Design review of the part built by this model. Coordinates are the model's own, in mm. Give positions to 0.01 mm unless a question says otherwise; leave off trailing zeros. Loops run counter-clockwise (first coordinate to the right, second up) from the corner with the lowest first, then second, coordinate; pieces in that order, holes last. Notation, with made-up numbers: (39, 77.5) -> (92, 77.5) arc R16 cw to (92, 102.5) -> close; hole circle Ø4 at (78.5, -28). An arc over 180 degrees is marked (long way). Answer as CSV lines item,"result".
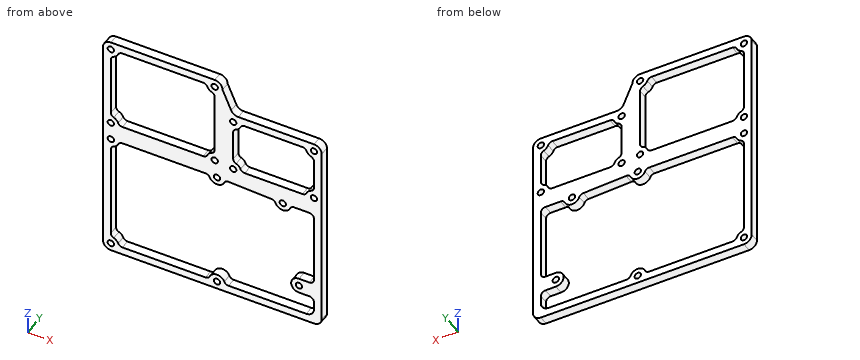
from build123d import *

# Parameters (mm, degrees)
SKETCH2_R                = 3.375
SKETCH2_R_2              = 1.375
PART_SCREWHOLES_DEPTH    = 4
PART_SCREWHOLES_2_DEPTH  = 4
PART_SCREWHOLES_3_DEPTH  = 4
PART_SCREWHOLES_4_DEPTH  = 4
PART_SCREWHOLES_5_DEPTH  = 4
PART_SCREWHOLES_6_DEPTH  = 4
PART_SCREWHOLES_7_DEPTH  = 4
PART_SCREWHOLES_8_DEPTH  = 4
PART_SCREWHOLES_9_DEPTH  = 4
PART_SCREWHOLES_10_DEPTH = 4
PART_SCREWHOLES_11_DEPTH = 4
PART_SCREWHOLES_12_DEPTH = 4
PART_SCREWHOLES_13_DEPTH = 4
PART_SCREWHOLES_14_DEPTH = 4
FRAME_START              = -4
SKETCH3_R                = 1.375
FRAME_DEPTH              = 4
GENERAL_ROUNDING_2MM_R   = 2


with BuildPart() as part:
    # Sketch2 → Part screwholes (new body)
    with BuildSketch(Plane(origin=(0, 0, 0), x_dir=(1, 0, 0), z_dir=(0, 1, 0))):
        with Locations(Location((-46, 51, 0), (0, 0, 270))):
            Circle(SKETCH2_R)
        with Locations(Location((-46, 51, 0), (0, 0, 270))):
            Circle(SKETCH2_R_2, mode=Mode.SUBTRACT)
    extrude(amount=PART_SCREWHOLES_DEPTH)



with BuildPart() as body_2:
    # Sketch2 → Part screwholes 2 (new body)
    with BuildSketch(Plane(origin=(0, 0, 0), x_dir=(1, 0, 0), z_dir=(0, 1, 0))):
        with Locations(Location((0, 51, 0), (0, 0, 270))):
            Circle(SKETCH2_R)
        with Locations(Location((0, 51, 0), (0, 0, 270))):
            Circle(SKETCH2_R_2, mode=Mode.SUBTRACT)
    extrude(amount=PART_SCREWHOLES_2_DEPTH)


with BuildPart() as body_3:
    # Sketch2 → Part screwholes 3 (new body)
    with BuildSketch(Plane(origin=(0, 0, 0), x_dir=(1, 0, 0), z_dir=(0, 1, 0))):
        with Locations(Location((0, 0, 0), (0, 0, 270))):
            Circle(SKETCH2_R)
        with Locations(Location((0, 0, 0), (0, 0, 270))):
            Circle(SKETCH2_R_2, mode=Mode.SUBTRACT)
    extrude(amount=PART_SCREWHOLES_3_DEPTH)


with BuildPart() as body_4:
    # Sketch2 → Part screwholes 4 (new body)
    with BuildSketch(Plane(origin=(0, 0, 0), x_dir=(1, 0, 0), z_dir=(0, 1, 0))):
        with Locations(Location((-46, 0, 0), (0, 0, 270))):
            Circle(SKETCH2_R)
        with Locations(Location((-46, 0, 0), (0, 0, 270))):
            Circle(SKETCH2_R_2, mode=Mode.SUBTRACT)
    extrude(amount=PART_SCREWHOLES_4_DEPTH)


with BuildPart() as body_5:
    # Sketch2 → Part screwholes 5 (new body)
    with BuildSketch(Plane(origin=(0, 0, 0), x_dir=(1, 0, 0), z_dir=(0, 1, 0))):
        with Locations(Location((-46, -8, 0), (0, 0, 270))):
            Circle(SKETCH2_R)
        with Locations(Location((-46, -8, 0), (0, 0, 270))):
            Circle(SKETCH2_R_2, mode=Mode.SUBTRACT)
    extrude(amount=PART_SCREWHOLES_5_DEPTH)


with BuildPart() as body_6:
    # Sketch2 → Part screwholes 6 (new body)
    with BuildSketch(Plane(origin=(0, 0, 0), x_dir=(1, 0, 0), z_dir=(0, 1, 0))):
        with Locations(Location((-1, -8, 0), (0, 0, 270))):
            Circle(SKETCH2_R)
        with Locations(Location((-1, -8, 0), (0, 0, 270))):
            Circle(SKETCH2_R_2, mode=Mode.SUBTRACT)
    extrude(amount=PART_SCREWHOLES_6_DEPTH)


with BuildPart() as body_7:
    # Sketch2 → Part screwholes 7 (new body)
    with BuildSketch(Plane(origin=(0, 0, 0), x_dir=(1, 0, 0), z_dir=(0, 1, 0))):
        with Locations(Location((7, -7, 0), (0, 0, 270))):
            Circle(SKETCH2_R)
        with Locations(Location((7, -7, 0), (0, 0, 270))):
            Circle(SKETCH2_R_2, mode=Mode.SUBTRACT)
    extrude(amount=PART_SCREWHOLES_7_DEPTH)


with BuildPart() as body_8:
    # Sketch2 → Part screwholes 8 (new body)
    with BuildSketch(Plane(origin=(0, 0, 0), x_dir=(1, 0, 0), z_dir=(0, 1, 0))):
        with Locations(Location((28.5, 1, 0), (0, 0, 270))):
            Circle(SKETCH2_R)
        with Locations(Location((28.5, 1, 0), (0, 0, 270))):
            Circle(SKETCH2_R_2, mode=Mode.SUBTRACT)
    extrude(amount=PART_SCREWHOLES_8_DEPTH)


with BuildPart() as body_9:
    # Sketch2 → Part screwholes 9 (new body)
    with BuildSketch(Plane(origin=(0, 0, 0), x_dir=(1, 0, 0), z_dir=(0, 1, 0))):
        with Locations(Location((35.5, 38.5, 0), (0, 0, 270))):
            Circle(SKETCH2_R)
        with Locations(Location((35.5, 38.5, 0), (0, 0, 270))):
            Circle(SKETCH2_R_2, mode=Mode.SUBTRACT)
    extrude(amount=PART_SCREWHOLES_9_DEPTH)


with BuildPart() as body_10:
    # Sketch2 → Part screwholes 10 (new body)
    with BuildSketch(Plane(origin=(0, 0, 0), x_dir=(1, 0, 0), z_dir=(0, 1, 0))):
        with Locations(Location((-1, -44, 0), (0, 0, 270))):
            Circle(SKETCH2_R)
        with Locations(Location((-1, -44, 0), (0, 0, 270))):
            Circle(SKETCH2_R_2, mode=Mode.SUBTRACT)
    extrude(amount=PART_SCREWHOLES_10_DEPTH)


with BuildPart() as body_11:
    # Sketch2 → Part screwholes 11 (new body)
    with BuildSketch(Plane(origin=(0, 0, 0), x_dir=(1, 0, 0), z_dir=(0, 1, 0))):
        with Locations(Location((-46, -44, 0), (0, 0, 270))):
            Circle(SKETCH2_R)
        with Locations(Location((-46, -44, 0), (0, 0, 270))):
            Circle(SKETCH2_R_2, mode=Mode.SUBTRACT)
    extrude(amount=PART_SCREWHOLES_11_DEPTH)


with BuildPart() as body_12:
    # Sketch2 → Part screwholes 12 (new body)
    with BuildSketch(Plane(origin=(0, 0, 0), x_dir=(1, 0, 0), z_dir=(0, 1, 0))):
        with Locations(Location((7, -30, 0), (0, 0, 270))):
            Circle(SKETCH2_R)
        with Locations(Location((7, -30, 0), (0, 0, 270))):
            Circle(SKETCH2_R_2, mode=Mode.SUBTRACT)
    extrude(amount=PART_SCREWHOLES_12_DEPTH)


with BuildPart() as body_13:
    # Sketch2 → Part screwholes 13 (new body)
    with BuildSketch(Plane(origin=(0, 0, 0), x_dir=(1, 0, 0), z_dir=(0, 1, 0))):
        with Locations(Location((42, -30, 0), (0, 0, 270))):
            Circle(SKETCH2_R)
        with Locations(Location((42, -30, 0), (0, 0, 270))):
            Circle(SKETCH2_R_2, mode=Mode.SUBTRACT)
    extrude(amount=PART_SCREWHOLES_13_DEPTH)


with BuildPart() as body_14:
    # Sketch2 → Part screwholes 14 (new body)
    with BuildSketch(Plane(origin=(0, 0, 0), x_dir=(1, 0, 0), z_dir=(0, 1, 0))):
        with Locations(Location((42, -7, 0), (0, 0, 270))):
            Circle(SKETCH2_R)
        with Locations(Location((42, -7, 0), (0, 0, 270))):
            Circle(SKETCH2_R_2, mode=Mode.SUBTRACT)
    extrude(amount=PART_SCREWHOLES_14_DEPTH)


with BuildPart() as part_1:
    add(part.part)

    add(body_2.part)  # Frame merges body 2

    add(body_3.part)  # Frame merges body 3

    add(body_4.part)  # Frame merges body 4

    add(body_5.part)  # Frame merges body 5

    add(body_6.part)  # Frame merges body 6

    add(body_7.part)  # Frame merges body 7

    add(body_8.part)  # Frame merges body 8

    add(body_9.part)  # Frame merges body 9

    add(body_10.part)  # Frame merges body 10

    add(body_11.part)  # Frame merges body 11

    add(body_12.part)  # Frame merges body 12

    add(body_13.part)  # Frame merges body 13

    add(body_14.part)  # Frame merges body 14
    # Sketch3 → Frame (add)
    with BuildSketch(Plane(origin=(0, 4, 0), x_dir=(1, 0, 0), z_dir=(0, 1, 0)).offset(FRAME_START)):
        with BuildLine():
            Line((-49.375, 51), (-49.375, -44))
            ThreePointArc((-49.375, -44), (-48.386485387, -46.386485387), (-46, -47.375))
            Line((-46, -47.375), (-1, -47.375))
            ThreePointArc((-1, -47.375), (1.386485387, -46.386485387), (2.375, -44))
            Line((2.375, -44), (6.117237342, -35.402968268))
            ThreePointArc((6.117237342, -35.402968268), (7.361851742, -33.927159489), (9.2117697, -33.375))
            Line((9.2117697, -33.375), (42, -33.375))
            ThreePointArc((42, -33.375), (44.386485387, -32.386485387), (45.375, -30))
            Line((45.375, -30), (45.375, 51))
            ThreePointArc((45.375, 51), (44.386485387, 53.386485387), (42, 54.375))
            Line((42, 54.375), (-46, 54.375))
            ThreePointArc((-46, 54.375), (-48.386485387, 53.386485387), (-49.375, 51))
        make_face()
        with Locations(Location((35.5, 38.5, 0), (0, 0, 270))):
            Circle(SKETCH3_R, mode=Mode.SUBTRACT)
        with Locations(Location((0, 51, 0), (0, 0, 270))):
            Circle(SKETCH3_R, mode=Mode.SUBTRACT)
        with Locations(Location((-46, 51, 0), (0, 0, 270))):
            Circle(SKETCH3_R, mode=Mode.SUBTRACT)
        with Locations(Location((-46, 0, 0), (0, 0, 270))):
            Circle(SKETCH3_R, mode=Mode.SUBTRACT)
        with Locations(Location((-46, -8, 0), (0, 0, 270))):
            Circle(SKETCH3_R, mode=Mode.SUBTRACT)
        with Locations(Location((0, 0, 0), (0, 0, 270))):
            Circle(SKETCH3_R, mode=Mode.SUBTRACT)
        with Locations(Location((-1, -8, 0), (0, 0, 270))):
            Circle(SKETCH3_R, mode=Mode.SUBTRACT)
        with Locations(Location((7, -7, 0), (0, 0, 270))):
            Circle(SKETCH3_R, mode=Mode.SUBTRACT)
        with Locations(Location((28.5, 1, 0), (0, 0, 270))):
            Circle(SKETCH3_R, mode=Mode.SUBTRACT)
        with Locations(Location((42, -7, 0), (0, 0, 270))):
            Circle(SKETCH3_R, mode=Mode.SUBTRACT)
        with Locations(Location((42, -30, 0), (0, 0, 270))):
            Circle(SKETCH3_R, mode=Mode.SUBTRACT)
        with Locations(Location((7, -30, 0), (0, 0, 270))):
            Circle(SKETCH3_R, mode=Mode.SUBTRACT)
        with Locations(Location((-46, -44, 0), (0, 0, 270))):
            Circle(SKETCH3_R, mode=Mode.SUBTRACT)
        with Locations(Location((-1, -44, 0), (0, 0, 270))):
            Circle(SKETCH3_R, mode=Mode.SUBTRACT)
        with BuildLine():
            Line((-46, 47.625), (-46, 3.375))
            ThreePointArc((-46, 3.375), (-43.613514613, 2.386485387), (-42.625, 0))
            Line((-42.625, 0), (-3.375, 0))
            ThreePointArc((-3.375, 0), (0, 3.375), (3.375, 0))
            Line((3.375, 0), (25.125, 1))
            ThreePointArc((25.125, 1), (28.5, 4.375), (31.875, 1))
            Line((31.875, 1), (42, 1))
            Line((42, 1), (42, 35.125))
            Line((42, 35.125), (35.5, 35.125))
            ThreePointArc((35.5, 35.125), (32.125, 38.5), (35.5, 41.875))
            Line((35.5, 41.875), (42, 41.875))
            Line((42, 41.875), (42, 47.625))
            ThreePointArc((42, 47.625), (41.011485387, 50.011485387), (38.625, 51))
            Line((38.625, 51), (3.375, 51))
            ThreePointArc((3.375, 51), (0, 47.625), (-3.375, 51))
            Line((-3.375, 51), (-42.625, 51))
            ThreePointArc((-42.625, 51), (-43.613514613, 48.613514613), (-46, 47.625))
        make_face(mode=Mode.SUBTRACT)
        with BuildLine():
            Line((-46, -11.375), (-46, -40.625))
            ThreePointArc((-46, -40.625), (-43.613514613, -41.613514613), (-42.625, -44))
            Line((-42.625, -44), (-4.375, -44))
            ThreePointArc((-4.375, -44), (-3.386485387, -41.613514613), (-1, -40.625))
            Line((-1, -40.625), (-1, -11.375))
            ThreePointArc((-1, -11.375), (-3.386485387, -10.386485387), (-4.375, -8))
            Line((-4.375, -8), (-42.625, -8))
            ThreePointArc((-42.625, -8), (-43.613514613, -10.386485387), (-46, -11.375))
        make_face(mode=Mode.SUBTRACT)
        with BuildLine():
            Line((10.375, -30), (38.625, -30))
            ThreePointArc((38.625, -30), (39.613514613, -27.613514613), (42, -26.625))
            Line((42, -26.625), (42, -10.375))
            ThreePointArc((42, -10.375), (39.613514613, -9.386485387), (38.625, -7))
            Line((38.625, -7), (10.375, -7))
            ThreePointArc((10.375, -7), (9.386485387, -9.386485387), (7, -10.375))
            Line((7, -10.375), (7, -26.625))
            ThreePointArc((7, -26.625), (9.386485387, -27.613514613), (10.375, -30))
        make_face(mode=Mode.SUBTRACT)
    extrude(amount=FRAME_DEPTH)

    # General rounding 2mm
    general_rounding_2mm_edges = [part_1.edges().sort_by_distance(p)[0] for p in [
        (-42.625, 2, 8),
        (-4.375, 2, 8),
        (-1, 2, 11.375),
        (-1, 2, 40.625),
        (-4.375, 2, 44),
        (-42.625, 2, 44),
        (-46, 2, 40.625),
        (-46, 2, 11.375),
        (42, 2, -35.125),
        (42, 2, -1),
        (31.875, 2, -1),
        (25.125, 2, -1),
        (3.375, 2, 0),
        (-3.375, 2, 0),
        (-42.625, 2, 0),
        (-46, 2, -3.375),
        (-46, 2, -47.625),
        (-42.625, 2, -51),
        (-3.375, 2, -51),
        (3.375, 2, -51),
        (42, 2, -41.875),
        (7, 2, 26.625),
        (7, 2, 10.375),
        (10.375, 2, 7),
        (38.625, 2, 7),
        (42, 2, 10.375),
        (42, 2, 26.625),
        (38.625, 2, 30),
        (10.375, 2, 30),
    ]]
    fillet(general_rounding_2mm_edges, radius=GENERAL_ROUNDING_2MM_R)


solid = part_1.part
Q1. We need section A-A, the plane z = 22. State the section outline as (x, y) points (3 decimals).
Filled sheet:
outline,"(-49.375, 0) -> (-46, 0) -> (-46, 4) -> (-49.375, 4) -> close; (-1, 0) -> (7, 0) -> (7, 4) -> (-1, 4) -> close; (42, 0) -> (45.375, 0) -> (45.375, 4) -> (42, 4) -> close"
Q2. Clearance check with flat-ended pins moving along their axes: pin 1 Ø1.2 at (x, y) = (27.5, 2) entering from +Z (3 decimals); pin 2 Ø12 at (x, z) = (-38.5, -22) entering from -Y. State where each tip first meets the part, or that it passes through.
Filled sheet:
pin 1,"stops at z = 33.375"
pin 2,"passes through"
Q3. We need section C-C, the plane y = 3.25. State how many separate pieces and enclosed holes the cut face has, and give its area (3 significant figures).
Filled sheet:
separate pieces,"1"
enclosed holes,"17"
area,"2,300 mm^2"
Q4. We need section D-D, the plane z = -38.5. State the section outline as (x, y) points (3 decimals), and give its area (3 significant figures).
Filled sheet:
outline,"(-49.375, 0) -> (-46, 0) -> (-46, 4) -> (-49.375, 4) -> close; (32.125, 0) -> (34.125, 0) -> (34.125, 4) -> (32.125, 4) -> close; (36.875, 0) -> (45.375, 0) -> (45.375, 4) -> (36.875, 4) -> close"
area,"55.5 mm^2"
Q5. To check wall thickness, follow probe 1 along Z at (x, y) = (-39, 3.2) (3 decimals); probe 2 along X at (y, z) = (1.2, 12) (3 decimals); probe 3 along X at (y, z) = (0.8, -19) (3 decimals). State the ranges of each line that lie inside material, in increasing order. Write a range as from..to.
Filled sheet:
probe 1,"z = -54.375..-51, 0..8, 44..47.375"
probe 2,"x = -49.375..-45.738, -1.262..7, 42..45.375"
probe 3,"x = -49.375..-46, 42..45.375"
Q6. We need section B-B, the plane z = -12. State the section outline as (x, y) points (3 decimals), and give its area (3 significant figures).
Filled sheet:
outline,"(-49.375, 0) -> (-46, 0) -> (-46, 4) -> (-49.375, 4) -> close; (42, 0) -> (45.375, 0) -> (45.375, 4) -> (42, 4) -> close"
area,"27.0 mm^2"
